from build123d import *

# Parameters (mm, degrees)
SKETCH1_R               = 56.75
BOSS_EXTRUDE3_DEPTH     = 23
SKETCH10_R              = 51.75
CUT_EXTRUDE3_DEPTH      = 18
SKETCH12_R              = 3.55
CUT_EXTRUDE4_DEPTH      = 83.250379938
SKETCH17_R              = 1.8
BOSS_EXTRUDE4_DEPTH     = 5.5
SKETCH18_R              = 1.8
BOSS_EXTRUDE5_DEPTH     = 5.5
FILLET5_R               = 1
FILLET6_R               = 1
CUT_EXTRUDE5_DEPTH      = 3
CUT_EXTRUDE5_DEPTH_BACK = 3
FILLET7_R               = 2
FILLET8_R               = 2
CHAMFER1_SIZE           = 4
CHAMFER1_SIZE2          = 2.309401077
SKETCH34_W              = 47.55
SKETCH34_H              = 5
BOSS_EXTRUDE6_DEPTH     = 29.515
SKETCH35_W              = 47.55
SKETCH35_H              = 5
BOSS_EXTRUDE7_DEPTH     = 29.515
CUT_EXTRUDE6_REACH      = 94.639
SKETCH42_R              = 2.34
CUT_EXTRUDE7_REACH      = 94.639
SKETCH43_R              = 2.34
CUT_EXTRUDE8_REACH      = 94.639
SKETCH44_R              = 2.34
CUT_EXTRUDE9_REACH      = 94.639
SKETCH45_R              = 2.34


with BuildPart() as part:
    # Sketch1 → Boss-Extrude3 (new body)
    with BuildSketch(Plane(origin=(0, 0, 0), x_dir=(1, 0, 0), z_dir=(0, 1, 0))):
        with Locations(Location((0, 0, 0), (0, 0, 270))):
            Circle(SKETCH1_R)
    extrude(amount=BOSS_EXTRUDE3_DEPTH)

    # Sketch10 → Cut-Extrude3 (cut)
    with BuildSketch(Plane(origin=(0, 23, 0), x_dir=(1, 0, 0), z_dir=(0, 1, 0))):
        with Locations(Location((0, 0, 0), (0, 0, 270))):
            Circle(SKETCH10_R)
    extrude(amount=-CUT_EXTRUDE3_DEPTH, mode=Mode.SUBTRACT)

    # Sketch12 → Cut-Extrude4 (cut, through all)
    with BuildSketch(Plane(origin=(0, 5, 0), x_dir=(1, 0, 0), z_dir=(0, 1, 0))):
        with Locations(Location((0, 0, 0), (0, 0, 270))):
            Circle(SKETCH12_R)
    extrude(amount=-CUT_EXTRUDE4_DEPTH, mode=Mode.SUBTRACT)

    # Sketch17 → Boss-Extrude4 (add)
    with BuildSketch(Plane(origin=(0, 5, 0), x_dir=(1, 0, 0), z_dir=(0, 1, 0))):
        with Locations(Location((-44.45, 0, 0), (0, 0, 270))):
            Circle(SKETCH17_R)
    extrude(amount=BOSS_EXTRUDE4_DEPTH)

    # Sketch18 → Boss-Extrude5 (add)
    with BuildSketch(Plane(origin=(0, 5, 0), x_dir=(1, 0, 0), z_dir=(0, 1, 0))):
        with Locations(Location((44.45, 0, 0), (0, 0, 270))):
            Circle(SKETCH18_R)
    extrude(amount=BOSS_EXTRUDE5_DEPTH)

    # Fillet5
    fillet5_edges = [part.edges().sort_by_distance(p)[0] for p in [
        (-44.45, 10.5, -1.8),
    ]]
    fillet(fillet5_edges, radius=FILLET5_R)

    # Fillet6
    fillet6_edges = [part.edges().sort_by_distance(p)[0] for p in [
        (44.45, 10.5, -1.8),
    ]]
    fillet(fillet6_edges, radius=FILLET6_R)

    # Sketch27 → Cut-Extrude5 (cut, two sides: drawn at the far end of the back side and taken through both)
    with BuildSketch(Plane.XY.offset(-54.25).offset(-CUT_EXTRUDE5_DEPTH_BACK)):
        with BuildLine():
            Line((7, 23), (7, 12))
            ThreePointArc((7, 12), (0, 5), (-7, 12))
            Line((-7, 12), (-7, 23))
            ThreePointArc((-7, 23), (0, 30), (7, 23))
        make_face()
    extrude(amount=CUT_EXTRUDE5_DEPTH + CUT_EXTRUDE5_DEPTH_BACK, mode=Mode.SUBTRACT)

    # Fillet7
    fillet7_edges = [part.edges().sort_by_distance(p)[0] for p in [
        (-51.630959196, 23, 3.508069632),
    ]]
    fillet(fillet7_edges, radius=FILLET7_R)

    # Fillet8
    fillet8_edges = [part.edges().sort_by_distance(p)[0] for p in [
        (-56.641553183, 23, 3.506701156),
    ]]
    fillet(fillet8_edges, radius=FILLET8_R)

    # Chamfer1
    chamfer1_edges = [part.edges().sort_by_distance(p)[0] for p in [
        (0, 0, -3.55),
    ]]
    chamfer1_side = [part.faces().sort_by_distance(p)[0] for p in [
        (0, 2.5, -3.55),
    ]]
    chamfer(chamfer1_edges, length=CHAMFER1_SIZE, length2=CHAMFER1_SIZE2, reference=chamfer1_side[0])

    # Sketch34 → Boss-Extrude6 (add)
    with BuildSketch(Plane(origin=(-40, 0, 0), x_dir=(0, 0, -1), z_dir=(1, 0, 0))):
        with Locations((0, 2.5)):
            Rectangle(SKETCH34_W, SKETCH34_H)
    extrude(amount=-BOSS_EXTRUDE6_DEPTH)

    # Sketch35 → Boss-Extrude7 (add)
    with BuildSketch(Plane(origin=(40, 0, 0), x_dir=(0, 0, -1), z_dir=(1, 0, 0))):
        with Locations((0, 2.5)):
            Rectangle(SKETCH35_W, SKETCH35_H)
    extrude(amount=BOSS_EXTRUDE7_DEPTH)

    # Sketch42 → Cut-Extrude6 (cut, up to next)
    with BuildSketch(Plane.XZ, mode=Mode.PRIVATE) as cut_extrude6_sk1:
        with Locations(Location((62.175, -12.435, 0), (0, 0, 270))):
            Circle(SKETCH42_R)
    cut_extrude6_tool1 = extrude(cut_extrude6_sk1.sketch, amount=-CUT_EXTRUDE6_REACH, mode=Mode.PRIVATE) & part.part
    add(cut_extrude6_tool1.solids().sort_by_distance((62.175, 0, -12.435))[0], mode=Mode.SUBTRACT)

    # Sketch43 → Cut-Extrude7 (cut, up to next)
    with BuildSketch(Plane(origin=(0, 0, 0), x_dir=(-1, 0, 0), z_dir=(0, -1, 0)), mode=Mode.PRIVATE) as cut_extrude7_sk1:
        with Locations(Location((-62.175, -12.435, 0), (0, 0, 90))):
            Circle(SKETCH43_R)
    cut_extrude7_tool1 = extrude(cut_extrude7_sk1.sketch, amount=-CUT_EXTRUDE7_REACH, mode=Mode.PRIVATE) & part.part
    add(cut_extrude7_tool1.solids().sort_by_distance((62.175, 0, 12.435))[0], mode=Mode.SUBTRACT)

    # Sketch44 → Cut-Extrude8 (cut, up to next)
    with BuildSketch(Plane(origin=(0, 0, 0), x_dir=(-1, 0, 0), z_dir=(0, -1, 0)), mode=Mode.PRIVATE) as cut_extrude8_sk1:
        with Locations(Location((62.175, 12.435, 0), (0, 0, 90))):
            Circle(SKETCH44_R)
    cut_extrude8_tool1 = extrude(cut_extrude8_sk1.sketch, amount=-CUT_EXTRUDE8_REACH, mode=Mode.PRIVATE) & part.part
    add(cut_extrude8_tool1.solids().sort_by_distance((-62.175, 0, -12.435))[0], mode=Mode.SUBTRACT)

    # Sketch45 → Cut-Extrude9 (cut, up to next)
    with BuildSketch(Plane(origin=(0, 0, 0), x_dir=(-1, 0, 0), z_dir=(0, -1, 0)), mode=Mode.PRIVATE) as cut_extrude9_sk1:
        with Locations(Location((62.175, -12.435, 0), (0, 0, 90))):
            Circle(SKETCH45_R)
    cut_extrude9_tool1 = extrude(cut_extrude9_sk1.sketch, amount=-CUT_EXTRUDE9_REACH, mode=Mode.PRIVATE) & part.part
    add(cut_extrude9_tool1.solids().sort_by_distance((-62.175, 0, 12.435))[0], mode=Mode.SUBTRACT)


solid = part.part
Verification items for the finished model (mm, model axes). A direction names the side the tool comes from. Coordinates: 2 decimals unless noted, no trailing zeros. Order: outer loops, then holes, each group sorted by start corner. A loop starts at its lowest first (then second) coordinate and runs counter-clockwise, first axis right, second up. Notation, with made-up numbers: (-19, 19.5) -> (-9, 19.5) arc R9 cw to (-9, 29.5) -> close; hole circle Ø9 at (-17.75, 89.5). An arc over 180 degrees is marked (long way). Put each result on its own line as item: value. Start each with the question number.
1. Material ranges on L1, parallel to Z at x = 57.5, y = 2 (3 decimals); L2, parallel to Y at x = -31, z = 5.5; L3, parallel to X at y = 10.75, z = 46.5, recorded low to high. Write a range as [from, to].
2. Access from +Z, -Z, +X, -X, +Y, -Y to the whole of each face (thin tool, end or side, straight path). Record for faces 5 (the flat face through (60, 2, -23.775)), 6 (the flat face through (60, 2, 23.775)), 7 (the cylindrical face through (0, 5, -54)).
3. Cross-section at A-A, the plane y = 18.25. Record the boundary of the cut face in (x, z).
4. Go/stop test with flat-tipped pins: pin 1 Ø5.5 at (x, z) = (0, 0) entering from +Y; pin 2 Ø2.5 at (x, y) = (-58, 2) entering from -Z (3 decimals); pin 3 Ø1 at (x, z) = (-16, -8) entering from +Y; pin 4 Ø2.5 at (x, y) = (63.5, 1.5) entering from +Z (3 decimals). Record where each tip stops, or that it passes through.
5. Mould release check, pull along X, two halves, no side actions. Record for faces 1 (the flat face through (62, 5, 0)), 2 (the cylindrical face through (17.05, 10.35, 54.13)), 3 (the cylindrical face through (42.693, 7.219, -0.39)), 4 (the flat face through (1, 5, 11)): released by +X, released by -X, zero draft, split by the parting line, or undercut.
Computed:
1. L1: [-23.775, 23.775]
1. L2: [0, 5]
1. L3: [-32.53, -22.71], [22.71, 32.53]
2. face 5: -Z, +X, +Y, -Y
2. face 6: +Z, +X, +Y, -Y
2. face 7: -Z, +Y
3. outline: (-7, -56.32) -> (-7, -51.27) arc R51.75 cw (long way) to (7, -51.27) -> (7, -56.32) arc R56.75 ccw (long way) to start
4. pin 1: through
4. pin 2: z = -23.775
4. pin 3: y = 5
4. pin 4: z = 23.775
5. face 1: zero draft
5. face 2: split by the parting line
5. face 3: undercut
5. face 4: undercut
